Design review of the part built by this model. Coordinates are the model's own, in mm. A direction names the side the tool comes from. Give positions to 0.01 mm unless a question says otherwise; leave off trailing zeros. Order: outer loops, then holes, each group sorted by start corner. A loop starts at its lowest first (then second) coordinate and runs counter-clockwise, first axis right, second up.
```python
from build123d import *

# Parameters (mm, degrees)
SKETCH1_W           = 180
SKETCH1_H           = 70
BOSS_EXTRUDE1_DEPTH = 3
SKETCH2_W           = 3
SKETCH2_H           = 27
SKETCH2_W_2         = 40
SKETCH2_H_2         = 3
CUT_EXTRUDE6_DEPTH  = 10


with BuildPart() as part:
    # Sketch1 → Boss-Extrude1 (new body)
    with BuildSketch(Plane(origin=(0, 0, 0), x_dir=(0, 0, -1), z_dir=(1, 0, 0))):
        Rectangle(SKETCH1_W, SKETCH1_H)
    extrude(amount=BOSS_EXTRUDE1_DEPTH)

    # Sketch2 → Cut-Extrude6 (cut)
    with BuildSketch(Plane(origin=(3, 0, 0), x_dir=(0, 0, -1), z_dir=(1, 0, 0))):
        Polygon((90, -32), (87, -32), (55, -32), (55, -35), (90, -35), align=None)
        with Locations((88.5, -18.5)):
            Rectangle(SKETCH2_W, SKETCH2_H)
        with Locations((25, -33.5)):
            Rectangle(SKETCH2_W_2, SKETCH2_H_2)
        with Locations((-25, -33.5)):
            Rectangle(SKETCH2_W_2, SKETCH2_H_2)
        Polygon((-55, -32), (-87, -32), (-90, -32), (-90, -35), (-55, -35), align=None)
        with Locations((-88.5, -18.5)):
            Rectangle(SKETCH2_W, SKETCH2_H)
        with Locations((-88.5, 18.5)):
            Rectangle(SKETCH2_W, SKETCH2_H)
        Polygon((-87, 32), (-55, 32), (-55, 35), (-90, 35), (-90, 32), align=None)
        with Locations((-25, 33.5)):
            Rectangle(SKETCH2_W_2, SKETCH2_H_2)
        with Locations((25, 33.5)):
            Rectangle(SKETCH2_W_2, SKETCH2_H_2)
        Polygon((55, 32), (87, 32), (90, 32), (90, 35), (55, 35), align=None)
        with Locations((88.5, 18.5)):
            Rectangle(SKETCH2_W, SKETCH2_H)
    extrude(amount=-CUT_EXTRUDE6_DEPTH, mode=Mode.SUBTRACT)


solid = part.part
```
1. Take a section at B-B (y = -17). State the section outline as (x, z) points.
Recorded:
outline: (0, -87) - (3, -87) - (3, 87) - (0, 87) - close
2. Draft analysis for pull direction Z (two halves, no side actions). For faces 5 (the face through (2, -19, -87)), 6 (the face through (2, 33, -5)), 7 (the face through (2, -34, 55)), state which applies: pulls with the +Z half, pulls with the -Z half, needs draft (parallel to the pull), parting line crosses it, or undercut.
Recorded:
face 5: pulls with the -Z half
face 6: undercut
face 7: pulls with the +Z half
3. Take a section at A-A (z = -17). State the section outline as (x, y) points, then the cut area to 3 significant figures.
Recorded:
outline: (0, -32) - (3, -32) - (3, 32) - (0, 32) - close
area: 192 mm2
4. For line 1 along Z through (x, y) = (1.45, -17); line 2 along Y through (x, z) = (2.8, 18), list the stretches that pass through material, from the lowest coordinate up.
Recorded:
line 1: z = -87 to 87
line 2: y = -32 to 32
5. For pin 1 (1.5 mm diameter, centred on x = 1, z = 13.5, fed in from -Y); pin 2 (1.5 mm diameter, centred on x = 2, y = 34, fed in from -Z); pin 3 (1.5 mm diameter, centred on x = 1, y = 21.5, fed in from -Z), all flat-tipped, find the tip position at first contact; note any pin that passes through.
Recorded:
pin 1: stops at y = -32
pin 2: stops at z = -55
pin 3: stops at z = -87
6. Machinability: for faces 1 (the face through (2, -34, 5)), 2 (the face through (2, -5, 89)), 3 (the face through (2, 5, 89)), 4 (the face through (2, 33, 5)), which of the approach directions +Z, -Z, +X, -X, +Y, -Y give a long, thin tool a straight path to every point of the face, cutting with its end or side? Answer none if there is none.
Recorded:
face 1: +X, -X, -Y
face 2: +Z, +X, -X, -Y
face 3: +Z, +X, -X, +Y
face 4: +X, -X, +Y
